Part model, mm, in its own coordinate system. A direction names the side the tool comes from. Round coordinates to 2 decimals unless told otherwise and drop trailing zeros. Write each loop counter-clockwise with the first axis right and the second up, starting at its lowest first coordinate (ties: lowest second). Pieces come first, ordered by that corner, then holes. Notation, with made-up numbers: M 10.25,-14 L 41.25,-14 A24 cw 41.25,16 Z; hole C 11.25,59.25 d4. An arc over 180 degrees is marked long. Answer as a JSON object with one key per item and string values. Group by question number.
1. Band-saw the part on B-B, the plane z = 3.75. Write the cut outline in (x, y), plus the area to 3 significant figures.
2. Band-saw the part on A-A, the plane z = 6.75. Write the cut outline in (x, y), plus the area to 3 significant figures.
3. Two-plate mould, pull along X, no slides. Class faces 1 (the face through (-16.38, 79.29, 0.99)), 2 (the face through (4.01, 91.293, 0.986)), 3 (the face through (-3.99, 91.297, 0.986)), 4 (the face through (-6, 82, 8)): +X half, -X half, draft (parallel to the pull), parting line (faces both ways), or undercut.
4. Drill centre lines: line 1 (X direction, y = 84, z = 4); line 2 (Y direction, x = -16, z = 1); line 3 (X direction, y = 81, z = 0.9). Where is each one in solid material? Low to high. Write a range as from..to.
5. Band-saw the part on C-C, the plane z = 0.5. Count the separate pieces of the cut face and the enclosed holes in it, plus the area to 3 significant figures.
6. Which spindle directions (+Z, -Z, +X, -X, +Y, -Y) get a long thin tool onto all of the face, cutting with end or side? Do faces 5 (the face through (0, 77, 6)), 6 (the face through (-3.25, 90, 4)), 7 (the face through (15.62, 79.29, 0.99)), 8 (the face through (2.075, 77.079, 0.74)). Say none if no direction does.
7. Drop flat-ended pins along their axis: pin 1 (3 mm diameter, centred on x = 12, z = 2, fed in from -Y); pin 2 (0.8 mm diameter, centred on y = 77, z = 7, fed in from -X); pin 3 (4 mm diameter, centred on y = 84, z = 6, fed in from +X); pin 4 (3 mm diameter, centred on x = -16, y = 81, fed in from +Z). Give the stop position or say it passes through.
from build123d import *

# Parameters (mm, degrees)
SKETCH1_R           = 1.75
BOSS_EXTRUDE1_DEPTH = 2
BOSS_EXTRUDE2_DEPTH = 6
SKETCH4_W           = 2
SKETCH4_H           = 1.583920217
CUT_EXTRUDE1_DEPTH  = 2
SKETCH5_R           = 2.75
CUT_EXTRUDE3_DEPTH  = 1.5


with BuildPart() as part:
    # Sketch1 → Boss-Extrude1 (new body)
    # profile 1 of 3: a face of its own
    with BuildSketch(Plane.XY):
        with BuildLine():
            ThreePointArc((-12.75, 81), (-13.657806533, 83.25313776), (-15.874079855, 84.247559717))
            add(Edge.make_bspline(
                [(-16, 84.25), (-15.936886934, 84.248565124), (-15.874079855, 84.247559717)],
                knots=[0, 0, 0, 0.007677399, 0.007677399, 0.007677399], degree=2))
            ThreePointArc((-16, 84.25), (-19.25, 81), (-16, 77.75))
            ThreePointArc((-16, 77.75), (-13.701902961, 78.701902961), (-12.75, 81))
        make_face()
        with Locations((-16, 81)):
            Circle(SKETCH1_R, mode=Mode.SUBTRACT)
    # profile 2 of 3: a face of its own
    with BuildSketch(Plane.XY):
        with BuildLine():
            ThreePointArc((6, 83.776937313), (-2.872281323, 78.509110436), (-3.25, 88.820497563))
            Line((-3.25, 88.820497563), (-3.25, 91.426937313))
            Line((-3.25, 91.426937313), (-4.75, 91.162446842))
            add(Edge.make_bspline(
                [(-15.874079855, 84.247559717), (-7.75611093, 84.117608401), (-4.75, 91.162446842)],
                knots=[0.007677399, 0.007677399, 0.007677399, 1, 1, 1], degree=2))
            ThreePointArc((-15.874079855, 84.247559717), (-13.657806533, 83.25313776), (-12.75, 81))
            ThreePointArc((-12.75, 81), (-13.701902961, 78.701902961), (-16, 77.75))
            add(Edge.make_bspline(
                [(-16, 77.75), (-8.124796889, 75.747320021), (0, 75.776937313)],
                knots=[0, 0, 0, 1, 1, 1], degree=2))
            add(Edge.make_bspline(
                [(16, 77.75), (8.124796889, 75.747320021), (0, 75.776937313)],
                knots=[0, 0, 0, 1, 1, 1], degree=2))
            ThreePointArc((16, 77.75), (12.750610128, 80.937028105), (15.874079855, 84.247559717))
            add(Edge.make_bspline(
                [(15.874079855, 84.247559717), (7.75611093, 84.117608401), (4.75, 91.162446842)],
                knots=[0.007677399, 0.007677399, 0.007677399, 1, 1, 1], degree=2))
            Line((4.75, 91.162446842), (3.25, 91.426937313))
            Line((3.25, 91.426937313), (3.25, 88.820497563))
            ThreePointArc((3.25, 88.820497563), (5.267826876, 86.649218636), (6, 83.776937313))
        make_face()
    # profile 3 of 3: a face of its own
    with BuildSketch(Plane.XY):
        with BuildLine():
            add(Edge.make_bspline(
                [(16, 84.25), (15.936886934, 84.248565124), (15.874079855, 84.247559717)],
                knots=[0, 0, 0, 0.007677399, 0.007677399, 0.007677399], degree=2))
            ThreePointArc((15.874079855, 84.247559717), (12.750610128, 80.937028105), (16, 77.75))
            ThreePointArc((16, 77.75), (18.298097039, 78.701902961), (19.25, 81))
            ThreePointArc((19.25, 81), (18.298097039, 83.298097039), (16, 84.25))
        make_face()
        with Locations((16, 81)):
            Circle(SKETCH1_R, mode=Mode.SUBTRACT)
    extrude(amount=BOSS_EXTRUDE1_DEPTH)

    # Sketch2 → Boss-Extrude2 (add)
    with BuildSketch(Plane.XY.offset(2)):
        with BuildLine():
            ThreePointArc((7.5, 83.776937313), (6.34921255, 87.769117168), (3.25, 90.53619023))
            Line((3.25, 90.53619023), (3.25, 88.820497563))
            ThreePointArc((3.25, 88.820497563), (5.267826876, 86.649218636), (6, 83.776937313))
            ThreePointArc((6, 83.776937313), (-2.872281323, 78.509110436), (-3.25, 88.820497563))
            Line((-3.25, 88.820497563), (-3.25, 90.53619023))
            ThreePointArc((-3.25, 90.53619023), (-3.992179856, 77.427724763), (7.5, 83.776937313))
        make_face()
    extrude(amount=BOSS_EXTRUDE2_DEPTH)

    # Sketch4 → Cut-Extrude1 (cut)
    with BuildSketch(Plane.XY.offset(8)):
        with Locations((0, 77.068897421)):
            Rectangle(SKETCH4_W, SKETCH4_H)
    extrude(amount=-CUT_EXTRUDE1_DEPTH, mode=Mode.SUBTRACT)

    # Sketch5 → Cut-Extrude3 (cut)
    with BuildSketch(Plane(origin=(0, 0, 0), x_dir=(-1, 0, 0), z_dir=(0, 0, -1))):
        with Locations((0, 75.274341128)):
            Circle(SKETCH5_R)
    extrude(amount=-CUT_EXTRUDE3_DEPTH, mode=Mode.SUBTRACT)


solid = part.part
Worked answers:
{
 "1": {"outline": "M -3.25,88.82 L -3.25,90.54 A7.5 ccw long 3.25,90.54 L 3.25,88.82 A6 cw long Z", "area": "53.4 mm^2"},
 "2": {"outline": "M -3.25,88.82 L -3.25,90.54 A7.5 ccw -1,76.34 L -1,77.86 A6 cw Z; M 1,76.34 A7.5 ccw 3.25,90.54 L 3.25,88.82 A6 cw 1,77.86 Z", "area": "50.4 mm^2"},
 "3": {"face 1": "undercut", "face 2": "+X half", "face 3": "-X half", "face 4": "draft"},
 "4": {"line 1": "x = -7.5..-6, 6..7.5", "line 2": "y = 77.75..79.25, 82.75..84.25", "line 3": "x = -19.25..-17.75, -14.25..-5.32, 5.32..14.25, 17.75..19.25"},
 "5": {"separate pieces": "2", "enclosed holes": "2", "area": "236 mm^2"},
 "6": {"face 5": "+Z, +Y, -Y", "face 6": "+Z, -Z, +Y", "face 7": "+Z, -Z", "face 8": "-Z, -Y"},
 "7": {"pin 1": "stops at y = 76.6", "pin 2": "stops at x = -3.95", "pin 3": "stops at x = 7.5", "pin 4": "passes through"}
}
